from build123d import *

# Parameters (mm, degrees)
SKETCH1_W           = 317.5
SKETCH1_H           = 559.70678
BOSS_EXTRUDE1_DEPTH = 3.175
SKETCH5_W           = 30.48
SKETCH5_H           = 22.86
CUT_EXTRUDE1_DEPTH  = 322.760101659
FILLET1_R           = 7.62
SKETCH5_3_W         = 241.3
SKETCH5_3_H         = 521.60678
CUT_EXTRUDE2_DEPTH  = 322.760101659


with BuildPart() as part:
    # Sketch1 → Boss-Extrude1 (new body)
    with BuildSketch(Plane.XY):
        Rectangle(SKETCH1_W, SKETCH1_H)
    extrude(amount=BOSS_EXTRUDE1_DEPTH)

    # Sketch5 → Cut-Extrude1 (cut, through all)
    with BuildSketch(Plane(origin=(0, 0, 0), x_dir=(-1, 0, 0), z_dir=(0, 0, -1))):
        with Locations((143.51, 216.35593)):
            Rectangle(SKETCH5_W, SKETCH5_H)
        with Locations((143.51, -123.82881)):
            Rectangle(SKETCH5_W, SKETCH5_H)
        with Locations((143.51, -225.42373)):
            Rectangle(SKETCH5_W, SKETCH5_H)
    cut_extrude1 = extrude(amount=-CUT_EXTRUDE1_DEPTH, mode=Mode.SUBTRACT)

    # Mirror1: Cut-Extrude1 across plane
    add(cut_extrude1.mirror(Plane(origin=(0, 0, 0), x_dir=(0, 0, 1), z_dir=(1, 0, 0))), mode=Mode.SUBTRACT)

    # Fillet1
    fillet1_edges = [part.edges().sort_by_distance(p)[0] for p in [
        (-128.27, 227.78593, 1.5875),
        (-158.75, 227.78593, 1.5875),
        (-158.75, 204.92593, 1.5875),
        (-128.27, 204.92593, 1.5875),
        (-128.27, -135.25881, 1.5875),
        (-128.27, -112.39881, 1.5875),
        (-158.75, -112.39881, 1.5875),
        (-158.75, -135.25881, 1.5875),
        (-128.27, -236.85373, 1.5875),
        (-128.27, -213.99373, 1.5875),
        (-158.75, -213.99373, 1.5875),
        (-158.75, -236.85373, 1.5875),
        (158.75, 227.78593, 1.5875),
        (128.27, 227.78593, 1.5875),
        (128.27, 204.92593, 1.5875),
        (158.75, 204.92593, 1.5875),
        (128.27, -112.39881, 1.5875),
        (128.27, -135.25881, 1.5875),
        (158.75, -135.25881, 1.5875),
        (158.75, -112.39881, 1.5875),
        (128.27, -213.99373, 1.5875),
        (128.27, -236.85373, 1.5875),
        (158.75, -236.85373, 1.5875),
        (158.75, -213.99373, 1.5875),
    ]]
    fillet(fillet1_edges, radius=FILLET1_R)

    # Sketch5<3> → Cut-Extrude2 (cut, through all)
    with BuildSketch(Plane(origin=(0, 0, 0), x_dir=(-1, 0, 0), z_dir=(0, 0, -1))):
        Rectangle(SKETCH5_3_W, SKETCH5_3_H)
    extrude(amount=-CUT_EXTRUDE2_DEPTH, mode=Mode.SUBTRACT)


solid = part.part
The listing builds one solid part. Answer for the finished solid, in the listing's coordinates (mm). Give positions to 0.01 mm unless a question says otherwise; leave off trailing zeros. Write each loop counter-clockwise with the first axis right and the second up, starting at its lowest first coordinate (ties: lowest second). Pieces come first, ordered by that corner, then holes.
Item 1: Section A-A, the plane y = 120.5 is taken. Write down the section's boundary in (x, z) (3 decimals).
Item 2: Find the intervals of material crossed by line 1 along X through (y, z) = (29, 1.9); line 2 along Y through (x, z) = (145.5, 1.2); line 3 along Y through (x, z) = (120.5, 1.5), in increasing order.
Item 3: Section B-B, the plane x = -11.5 is taken. Write down the section's boundary in (y, z) (3 decimals), plus the area to 3 significant figures.
Item 4: Flat-ended cylindrical pins translate along their axes: P1, Ø1, axis at y = 214.5, z = 1.5, coming from the -X side; P2, Ø1.6, axis at y = -125, z = 1, coming from the +X side. Find the tip coordinate at first contact, or state that the pin passes through.
Completed:
1. outline: (-158.75, 0) - (-120.65, 0) - (-120.65, 3.175) - (-158.75, 3.175) - close; (120.65, 0) - (158.75, 0) - (158.75, 3.175) - (120.65, 3.175) - close
2. line 1: x = -158.75 to -120.65, 120.65 to 158.75
2. line 2: y = -279.85 to -236.85, -213.99 to -135.26, -112.4 to 204.93, 227.79 to 279.85
2. line 3: y = -279.85 to -260.8, 260.8 to 279.85
3. outline: (-279.853, 0) - (-260.803, 0) - (-260.803, 3.175) - (-279.853, 3.175) - close; (260.803, 0) - (279.853, 0) - (279.853, 3.175) - (260.803, 3.175) - close
3. area: 121 mm2
4. P1: stops at x = -128.27
4. P2: stops at x = 128.27
